from build123d import *

# Parameters (mm, degrees)
SKETCH1_R             = 11.176
BOSS_EXTRUDE1_DEPTH   = 19.05
BOSS_EXTRUDE1_2_DEPTH = 19.05
BOSS_EXTRUDE2_DEPTH   = 50.8
BOSS_EXTRUDE3_DEPTH   = 31.75
SKETCH1_5_R           = 11.176
SKETCH1_5_R_2         = 6.35
BOSS_EXTRUDE4_DEPTH   = 12.7


with BuildPart() as part:
    # Sketch1 → Boss-Extrude1 (new body)
    with BuildSketch(Plane(origin=(0, 0, 0), x_dir=(1, 0, 0), z_dir=(0, 1, 0))):
        with BuildLine():
            ThreePointArc((-63.02104825, 25.4), (-88.42104825, 0), (-63.02104825, -25.4))
            Line((-63.02104825, -25.4), (-18.57104825, -25.4))
            ThreePointArc((-18.57104825, -25.4), (-43.97104825, -1.3e-08), (-18.571048276, 25.4))
            Line((-18.571048276, 25.4), (-63.02104825, 25.4))
        make_face()
        with Locations(Location((-63.02104825, 0, 0), (0, 0, 90))):
            Circle(SKETCH1_R, mode=Mode.SUBTRACT)
    extrude(amount=BOSS_EXTRUDE1_DEPTH)



with BuildPart() as body_2:
    # Sketch1 → Boss-Extrude1 2 (new body)
    with BuildSketch(Plane(origin=(0, 0, 0), x_dir=(1, 0, 0), z_dir=(0, 1, 0))):
        with BuildLine():
            ThreePointArc((-18.571048276, 25.4), (6.82895175, 1.3e-08), (-18.57104825, -25.4))
            Line((-18.57104825, -25.4), (25.87895175, -25.4))
            ThreePointArc((25.87895175, -25.4), (51.27895175, 0), (25.87895175, 25.4))
            Line((25.87895175, 25.4), (-18.571048276, 25.4))
        make_face()
        with Locations(Location((25.87895175, 0, 0), (0, 0, 90))):
            Circle(SKETCH1_R, mode=Mode.SUBTRACT)
    extrude(amount=BOSS_EXTRUDE1_2_DEPTH)


with BuildPart() as part_1:
    add(part.part)

    add(body_2.part)  # Boss-Extrude2 merges body 2
    # Sketch1<3> → Boss-Extrude2 (add)
    with BuildSketch(Plane(origin=(0, 0, 0), x_dir=(1, 0, 0), z_dir=(0, 1, 0))):
        with BuildLine():
            Line((-24.92104825, 12.869681465), (-24.92104825, 24.593444248))
            ThreePointArc((-24.92104825, 24.593444248), (-36.531560492, 17.960512242), (-43.164492498, 6.35))
            Line((-43.164492498, 6.35), (-31.440729714, 6.35))
            ThreePointArc((-31.440729714, 6.35), (-28.718737667, 10.147689417), (-24.92104825, 12.869681465))
        make_face()
        with BuildLine():
            ThreePointArc((6.022395999, 6.35), (-0.610536008, 17.960512242), (-12.22104825, 24.593444248))
            Line((-12.22104825, 24.593444248), (-12.22104825, 12.869681465))
            ThreePointArc((-12.22104825, 12.869681465), (-8.423358833, 10.147689417), (-5.701366785, 6.35))
            Line((-5.701366785, 6.35), (6.022395999, 6.35))
        make_face()
        with BuildLine():
            ThreePointArc((-43.164492498, -6.35), (-36.531560492, -17.960512242), (-24.92104825, -24.593444248))
            Line((-24.92104825, -24.593444248), (-24.92104825, -12.869681465))
            ThreePointArc((-24.92104825, -12.869681465), (-28.718737667, -10.147689417), (-31.440729714, -6.35))
            Line((-31.440729714, -6.35), (-43.164492498, -6.35))
        make_face()
        with BuildLine():
            Line((-12.22104825, -12.869681465), (-12.22104825, -24.593444248))
            ThreePointArc((-12.22104825, -24.593444248), (-0.610536008, -17.960512242), (6.022395999, -6.35))
            Line((6.022395999, -6.35), (-5.701366785, -6.35))
            ThreePointArc((-5.701366785, -6.35), (-8.423358833, -10.147689417), (-12.22104825, -12.869681465))
        make_face()
    extrude(amount=BOSS_EXTRUDE2_DEPTH)

    # Sketch1<4> → Boss-Extrude3 (add)
    with BuildSketch(Plane(origin=(0, 0, 0), x_dir=(1, 0, 0), z_dir=(0, 1, 0))):
        with BuildLine():
            ThreePointArc((-18.571048276, 25.4), (-21.771557292, 25.197554284), (-24.92104825, 24.593444248))
            Line((-24.92104825, 24.593444248), (-24.92104825, 12.869681465))
            ThreePointArc((-24.92104825, 12.869681465), (-18.57104825, 14.351), (-12.22104825, 12.869681465))
            Line((-12.22104825, 12.869681465), (-12.22104825, 24.593444248))
            ThreePointArc((-12.22104825, 24.593444248), (-15.370539234, 25.197554287), (-18.571048276, 25.4))
        make_face()
        with BuildLine():
            Line((-24.92104825, -12.869681465), (-24.92104825, -24.593444248))
            ThreePointArc((-24.92104825, -24.593444248), (-21.771557279, -25.197554285), (-18.57104825, -25.4))
            ThreePointArc((-18.57104825, -25.4), (-15.370539221, -25.197554285), (-12.22104825, -24.593444248))
            Line((-12.22104825, -24.593444248), (-12.22104825, -12.869681465))
            ThreePointArc((-12.22104825, -12.869681465), (-18.57104825, -14.351), (-24.92104825, -12.869681465))
        make_face()
        with BuildLine():
            ThreePointArc((-43.164492498, 6.35), (-43.768602535, 3.200509029), (-43.97104825, 0))
            Line((-43.97104825, 0), (-32.92204825, 0))
            ThreePointArc((-32.92204825, 0), (-32.546812982, 3.260245566), (-31.440729714, 6.35))
            Line((-31.440729714, 6.35), (-43.164492498, 6.35))
        make_face()
        with BuildLine():
            ThreePointArc((-5.701366785, 6.35), (-4.595283518, 3.260245566), (-4.22004825, 0))
            Line((-4.22004825, 0), (6.82895175, 0))
            ThreePointArc((6.82895175, 0), (6.626506035, 3.200509029), (6.022395999, 6.35))
            Line((6.022395999, 6.35), (-5.701366785, 6.35))
        make_face()
        with BuildLine():
            Line((-32.92204825, 0), (-43.97104825, 0))
            ThreePointArc((-43.97104825, 0), (-43.768602535, -3.200509029), (-43.164492498, -6.35))
            Line((-43.164492498, -6.35), (-31.440729714, -6.35))
            ThreePointArc((-31.440729714, -6.35), (-32.546812982, -3.260245566), (-32.92204825, 0))
        make_face()
        with BuildLine():
            Line((6.82895175, 0), (-4.22004825, 0))
            ThreePointArc((-4.22004825, 0), (-4.595283518, -3.260245566), (-5.701366785, -6.35))
            Line((-5.701366785, -6.35), (6.022395999, -6.35))
            ThreePointArc((6.022395999, -6.35), (6.626506035, -3.200509029), (6.82895175, 0))
        make_face()
    extrude(amount=BOSS_EXTRUDE3_DEPTH)

    # Sketch1<5> → Boss-Extrude4 (add)
    # profile 1 of 2: a face of its own
    with BuildSketch(Plane(origin=(0, 0, 0), x_dir=(1, 0, 0), z_dir=(0, 1, 0))):
        with Locations(Location((-63.02104825, 0, 0), (0, 0, 90))):
            Circle(SKETCH1_5_R)
        with Locations(Location((-63.02104825, 0, 0), (0, 0, 270))):
            Circle(SKETCH1_5_R_2, mode=Mode.SUBTRACT)
    # profile 2 of 2: a face of its own
    with BuildSketch(Plane(origin=(0, 0, 0), x_dir=(1, 0, 0), z_dir=(0, 1, 0))):
        with Locations(Location((25.87895175, 0, 0), (0, 0, 90))):
            Circle(SKETCH1_5_R)
        with Locations(Location((25.87895175, 0, 0), (0, 0, 270))):
            Circle(SKETCH1_5_R_2, mode=Mode.SUBTRACT)
    extrude(amount=BOSS_EXTRUDE4_DEPTH)


solid = part_1.part
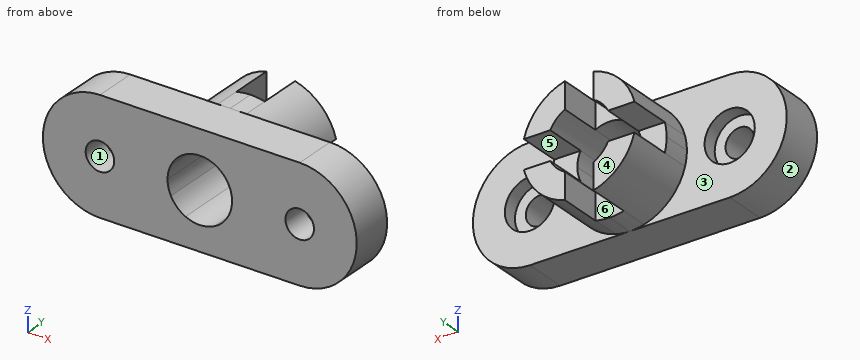
The model under review builds one solid part; all positions refer to its coordinate system, in mm. Face numbers are marked on the shaded views. A direction names the side the tool comes from. Give positions to 0.01 mm unless a question says otherwise; leave off trailing zeros. Order: outer loops, then holes, each group sorted by start corner. A loop starts at its lowest first (then second) coordinate and runs counter-clockwise, first axis right, second up. Notation, with made-up numbers: M 48,69 L 71,69 A19 cw 71,81 Z; hole C 45,73.5 d11. An arc over 180 degrees is marked long. One line per question, with ' | ' between items. Start each with the question number.
1) Consider section D-D, the plane z = 5. Give the boundary of the cut face in (x, y).
2) Wall thickness on L1, parallel to Y at x = -58.5, z = -22; L2, parallel to X at y = 33, z = 9; L3, parallel to X at y = 7.5, z = -7.5: over which ranges is each line inside the solid? List them lowest first. Write a range as from..to.
3) Consider section C-C, the plane x = -66. Give the boundary of the cut face in (y, z).
4) Consider section A-A, the plane y = 29.5. Give the boundary of the cut face in (x, z), then the cut area to 3 significant figures.
5) Consider section B-B, the plane y = 14. Give the boundary of the cut face in (x, z), then the cut area to 3 significant figures.
6) Mouldability with a two-part tool opening along X and no side actions: class the marked faces 1, 2 and 3 as pulls with the +X half, pulls with the -X half, needs draft (parallel to the pull), parting line crosses it, or undercut.
7) For the marked faces 4, 5 and 6, list the 3-axis set-ups (+Z, -Z, +X, -X, +Y, -Y) from which the entire face can be reached by the end or side of a thin tool; tool diameter is ignored.
8) Clearance check with flat-ended pins moving along their axes: P1, Ø9.5, axis at x = -0.5, y = 37.5, coming from the +Z side; P2, Ø11, axis at x = -66, z = -4, coming from the +Y side; P3, Ø3.5, axis at y = 43, z = 16.5, coming from the +X side. State where each tip first meets the part, or that it passes through.
Found:
1) outline: M -87.92,0 L -66.94,0 L -66.94,12.7 L -73.02,12.7 L -73.02,19.05 L -87.92,19.05 Z; M -59.11,0 L -32.02,0 L -32.02,31.75 L -43.47,31.75 L -43.47,19.05 L -53.03,19.05 L -53.03,12.7 L -59.11,12.7 Z; M -5.12,0 L 21.96,0 L 21.96,12.7 L 15.88,12.7 L 15.88,19.05 L 6.33,19.05 L 6.33,31.75 L -5.12,31.75 Z; M 29.79,0 L 50.78,0 L 50.78,19.05 L 35.87,19.05 L 35.87,12.7 L 29.79,12.7 Z
2) L1: y = 0..19.05 | L2: x = -42.32..-29.75, -7.39..5.18 | L3: x = -87.29..-30.81, -6.34..50.15
3) outline: M 0,-25.22 L 19.05,-25.22 L 19.05,-10.77 L 12.7,-10.77 L 12.7,-5.61 L 0,-5.61 Z; M 0,5.61 L 12.7,5.61 L 12.7,10.77 L 19.05,10.77 L 19.05,25.22 L 0,25.22 Z
4) outline: C -18.57,0 d50.8; hole C -18.57,0 d28.7 | area: 1,380 mm²
5) outline: M -63.02,-25.4 L 25.88,-25.4 A25.4 ccw 25.88,25.4 L -63.02,25.4 A25.4 ccw Z; hole C -63.02,0 d22.35; hole C -18.57,0 d28.7; hole C 25.88,0 d22.35 | area: 5,110 mm²
6) face 1: undercut | face 2: pulls with the -X half | face 3: needs draft
7) face 4: +Z, -Z, +X, -X, +Y | face 5: +X, -X, +Y | face 6: +Z, -Z, +Y
8) P1: stops at z = 21.63 | P2: stops at y = 12.7 | P3: stops at x = 2.11
